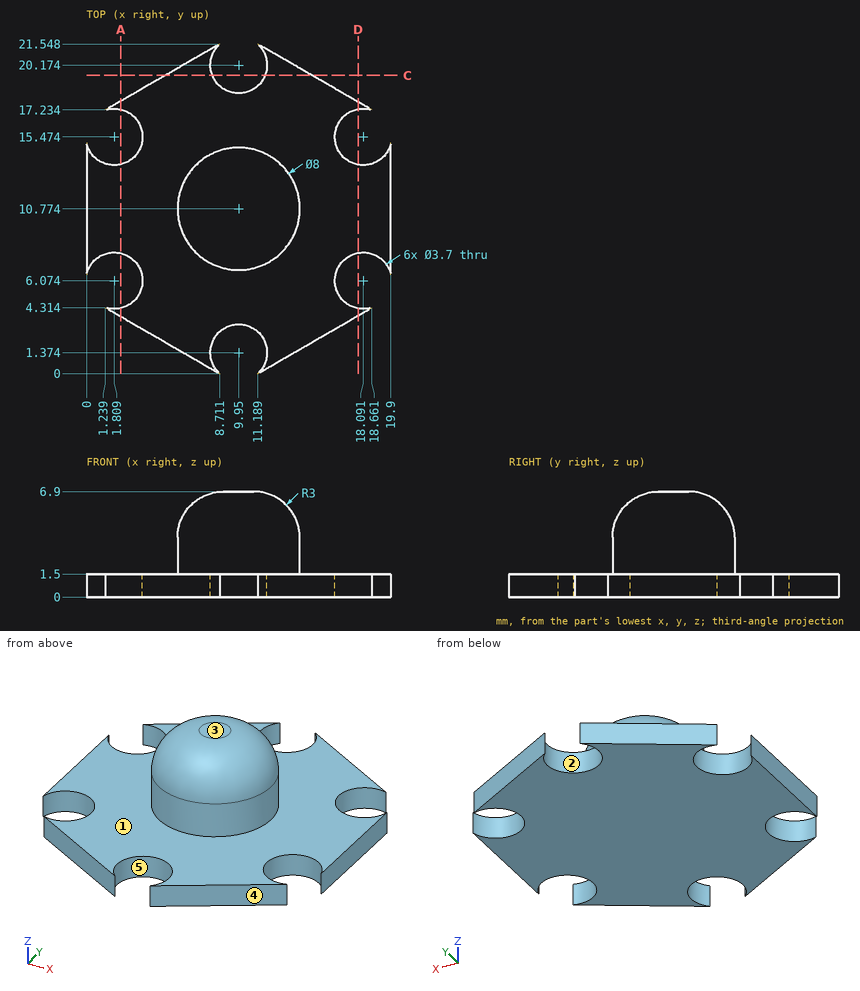
Drawing for the job (mm, zero at the part's lowest x, y, z). A direction names the side the tool comes from. Give positions to 0.01 mm unless a question says otherwise; leave off trailing zeros. Loops run counter-clockwise (first coordinate to the right, second up) from the corner with the lowest first, then second, coordinate; pieces in that order, holes last.
1) 3-axis set-ups, long thin cutter, end or side, ignore diameter. For the marked faces 1 and 2: which of +Z, -Z, +X, -X, +Y, -Y reach the whole face in a straight line?
Values follow:
face 1: +Z
face 2: +Z, -Z
2) Probe line 1 along X through (y, z) = (14.25, 0.5) (1 decimal); line 2 along Y through (x, z) = (3.25, 1) (1 decimal); line 3 along Y through (x, z) = (9.95, 0.35). List the from-to ranges inside material, lowest first.
Values follow:
line 1: x = 0 to 0.4, 3.2 to 16.7, 19.5 to 19.9
line 2: y = 3.2 to 4.9, 7.2 to 14.3, 16.6 to 18.4
line 3: y = 3.22 to 18.32
3) Drop flat-ended pins along their axis: P1, Ø3, axis at x = 9.95, y = 20.17, coming from the -Z side; P2, Ø4, axis at x = 16.5, z = 2, coming from the +Y side; P3, Ø2, axis at x = 15.5, y = 7.5, coming from the +Z side; P4, Ø3, axis at x = 10, y = 5.5, coming from the +Z side. Give the stop position or say it passes through.
Values follow:
P1: passes through
P2: stops at y = 19.6
P3: stops at z = 1.5
P4: stops at z = 5.04
4) Band-saw the part on C-C on y = 19.5. List the corners of the cut face in (x, z).
Values follow:
outline: (5.16, 0) - (8.23, 0) - (8.23, 1.5) - (5.16, 1.5) - close; (11.67, 0) - (14.74, 0) - (14.74, 1.5) - (11.67, 1.5) - close
5) Band-saw the part on D-D on x = 17.75. List the corners of the cut face in (y, z).
Values follow:
outline: (3.79, 0) - (4.26, 0) - (4.26, 1.5) - (3.79, 1.5) - close; (7.89, 0) - (13.66, 0) - (13.66, 1.5) - (7.89, 1.5) - close; (17.29, 0) - (17.76, 0) - (17.76, 1.5) - (17.29, 1.5) - close
6) Band-saw the part on A-A on x = 2.25. List the corners of the cut face in (y, z).
Values follow:
outline: (3.73, 0) - (4.28, 0) - (4.28, 1.5) - (3.73, 1.5) - close; (7.87, 0) - (13.68, 0) - (13.68, 1.5) - (7.87, 1.5) - close; (17.27, 0) - (17.82, 0) - (17.82, 1.5) - (17.27, 1.5) - close
7) Two-plate mould, pull along Y, no slides. Class the marked faces 3, 4 and 5: released by +Y, released by -Y, zero draft, split by the parting line, or undercut.
Values follow:
face 3: zero draft
face 4: released by -Y
face 5: undercut
